```python
from build123d import *

# Parameters (mm, degrees)
ESQUISSE1_W             = 33
ESQUISSE1_H             = 60
BOSS_EXTRU_1_DEPTH      = 3
ESQUISSE3_R             = 3.75
BOSS_EXTRU_2_DEPTH      = 1.2
ESQUISSE4_R             = 1.75
ENL_V_MAT_EXTRU_1_DEPTH = 69.541957953


with BuildPart() as part:
    # Esquisse1 → Boss.-Extru.1 (new body)
    with BuildSketch(Plane.XY):
        with Locations((16.5, 30)):
            Rectangle(ESQUISSE1_W, ESQUISSE1_H)
    extrude(amount=BOSS_EXTRU_1_DEPTH)

    # Esquisse3 → Boss.-Extru.2 (add)
    with BuildSketch(Plane(origin=(0, 0, 0), x_dir=(-1, 0, 0), z_dir=(0, 0, -1))):
        with Locations((-3.75, 53)):
            Circle(ESQUISSE3_R)
        with Locations((-3.75, 7)):
            Circle(ESQUISSE3_R)
    extrude(amount=BOSS_EXTRU_2_DEPTH)

    # Esquisse4 → Enlèv. mat.-Extru.1 (cut, through all)
    with BuildSketch(Plane(origin=(0, 0, 0), x_dir=(-1, 0, 0), z_dir=(0, 0, -1))):
        with Locations((-28.75, 40)):
            Circle(ESQUISSE4_R)
        with Locations((-28.75, 20)):
            Circle(ESQUISSE4_R)
    extrude(amount=-ENL_V_MAT_EXTRU_1_DEPTH, mode=Mode.SUBTRACT)


solid = part.part
```
Here's how the part is built. I have some questions about the finished solid (model axes, mm). A direction names the side the tool comes from. Coordinates: 2 decimals unless noted, no trailing zeros. Loops run counter-clockwise (first coordinate to the right, second up) from the corner with the lowest first, then second, coordinate; pieces in that order, holes last. Notation, with made-up numbers: (59, -36) - (115, -36) arc R5 cw to (115, -27) - close; hole circle Ø5 at (68.25, -15). An arc over 180 degrees is marked (long way). Return JSON: item names as keys, results as strings. Group by question number.
Item 1: If we section it at C-C on x = 3.75: Write out the boundary of the cut face in (y, z), and give its area (3 significant figures).
Item 2: We'd pull the mould along Y, two halves only. Please class faces 3 (the face through (16, 30, 0)), 4 (the face through (16, 0, 1)), 5 (the face through (4, 7, -1.2)): +Y half, -Y half, draft (parallel to the pull), parting line (faces both ways), or undercut.
Item 3: If we section it at A-A on x = 28.75: Write out the boundary of the cut face in (y, z), and give its area (3 significant figures).
Item 4: I need wall thicknesses on line 1 (Y direction, x = 28.75, z = 0.95); line 2 (Z direction, x = 12, y = 15); line 3 (Y direction, x = 5, z = -0.5). Which ranges of each line are inside material? Lowest first, please. Write a range as from..to.
Item 5: If we section it at D-D on y = 55.5: Write out the boundary of the cut face in (x, z), and give its area (3 significant figures).
Item 6: On a 3-axis mill with a long thin cutter (end or side, diameter ignored), from which of +Z, -Z, +X, -X, +Y, -Y can I reach the whole of each face in a straight line? I mean faces 1 (the face through (30.04, 21.18, 1.48)), 2 (the face through (4.56, 49.34, -0.59)). Say none if no direction works.
Item 7: Will this pin go through, and if not, where does the flat tip stop? P1, Ø10, axis at x = 25, y = 30, coming from the -Z side.
Item 8: If we section it at B-B on y = 20: Write out the boundary of the cut face in (x, z), and give its area (3 significant figures).
Calculated:
{
 "1": {"outline": "(0, 0) - (3.25, 0) - (3.25, -1.2) - (10.75, -1.2) - (10.75, 0) - (49.25, 0) - (49.25, -1.2) - (56.75, -1.2) - (56.75, 0) - (60, 0) - (60, 3) - (0, 3) - close", "area": "198 mm^2"},
 "2": {"face 3": "undercut", "face 4": "-Y half", "face 5": "draft"},
 "3": {"outline": "(0, 0) - (18.25, 0) - (18.25, 3) - (0, 3) - close; (21.75, 0) - (38.25, 0) - (38.25, 3) - (21.75, 3) - close; (41.75, 0) - (60, 0) - (60, 3) - (41.75, 3) - close", "area": "159 mm^2"},
 "4": {"line 1": "y = 0..18.25, 21.75..38.25, 41.75..60", "line 2": "z = 0..3", "line 3": "y = 3.46..10.54, 49.46..56.54"},
 "5": {"outline": "(0, 0) - (0.95, 0) - (0.95, -1.2) - (6.55, -1.2) - (6.55, 0) - (33, 0) - (33, 3) - (0, 3) - close", "area": "106 mm^2"},
 "6": {"face 1": "+Z, -Z", "face 2": "-Z"},
 "7": {"P1": "stops at z = 0"},
 "8": {"outline": "(0, 0) - (27, 0) - (27, 3) - (0, 3) - close; (30.5, 0) - (33, 0) - (33, 3) - (30.5, 3) - close", "area": "88.5 mm^2"}
}
